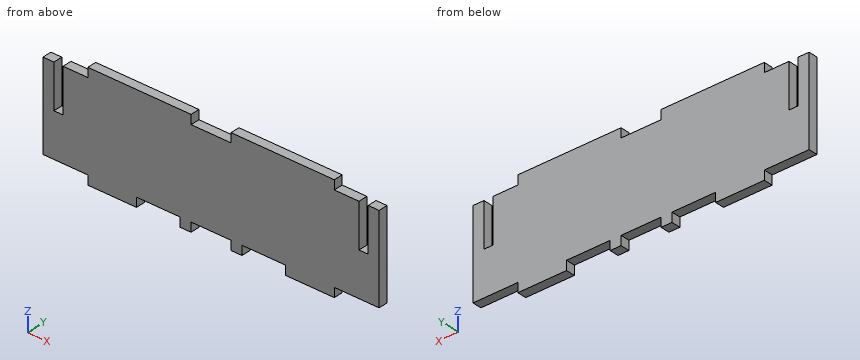
```python
from build123d import *

# Parameters (mm, degrees)
F0_W     = 60.071
F0_H     = 5.334
F0_W_2   = 28.321
F0_W_3   = 6.35
F1_DEPTH = 5.3594


with BuildPart() as f1:
    # F0 (on Front) → F1 (new body)
    with BuildSketch(Plane.XZ):
        with Locations((56.1213, 53.467)):
            Rectangle(F0_W, F0_H)
        with Locations((139.466246, 53.467)):
            Rectangle(F0_W, F0_H)
        Polygon((0, 50.8), (0, 0), (26.0858, 0), (54.4068, 0), (79.8068, 0), (86.1568, 0), (109.430746, 0), (115.780746, 0), (141.180746, 0), (169.501746, 0), (195.587546, 0), (195.587546, 50.8), (189.237546, 50.8), (189.237546, 25.4), (183.903546, 25.4), (183.903546, 50.8), (169.501746, 50.8), (109.430746, 50.8), (86.1568, 50.8), (26.0858, 50.8), (11.684, 50.8), (11.684, 25.4), (6.35, 25.4), (6.35, 50.8), align=None)
        with Locations((40.2463, -2.667)):
            Rectangle(F0_W_2, F0_H)
        with Locations((82.9818, -2.667)):
            Rectangle(F0_W_3, F0_H)
        with Locations((112.605746, -2.667)):
            Rectangle(F0_W_3, F0_H)
        with Locations((155.341246, -2.667)):
            Rectangle(F0_W_2, F0_H)
    extrude(amount=F1_DEPTH)


solid = f1.part
```
The model under review builds one solid part; all positions refer to its coordinate system, in mm. Round coordinates to 2 decimals unless told otherwise and drop trailing zeros. Loops run counter-clockwise (first coordinate to the right, second up) from the corner with the lowest first, then second, coordinate; pieces in that order, holes last. Notation, with made-up numbers: (7.5, -17) - (63.5, -17) arc R24 ccw to (63.5, 1) - close; hole circle Ø2 at (36, 3). An arc over 180 degrees is marked (long way). Write each question's results on one line, items separated by ' | '. Start each with the question number.
Q1. Take a section at A-A on z = 44. Give the boundary of the cut face in (x, y), plus the area to 3 significant figures.
Q2. Wall thickness on line 1 along X through (y, z) = (-0.9, -1); line 2 along X through (y, z) = (-4.8, 48.5); line 3 along Z through (x, y) = (179, -1.45): over which ranges is each line inside the solid? List them lowest first. Write a range as [from, to].
Q3. Take a section at B-B on x = 62. Give the boundary of the cut face in (y, z).
Q4. Insertion check: P1, Ø2.5, axis at x = 69.5, y = -2, coming from the -Z side; P2, Ø1.6, axis at x = 99.5, y = -2, coming from the +Z side; P3, Ø2.5, axis at y = -2, z = 53.5, coming from the -X side. Each pin has a flat end and moves straight along its axis. Give the tip position at first contact, or say it passes through.
Data:
1) outline: (0, -5.36) - (6.35, -5.36) - (6.35, 0) - (0, 0) - close; (11.68, -5.36) - (183.9, -5.36) - (183.9, 0) - (11.68, 0) - close; (189.24, -5.36) - (195.59, -5.36) - (195.59, 0) - (189.24, 0) - close | area: 991 mm²
2) line 1: x = [26.09, 54.41], [79.81, 86.16], [109.43, 115.78], [141.18, 169.5] | line 2: x = [0, 6.35], [11.68, 183.9], [189.24, 195.59] | line 3: z = [0, 50.8]
3) outline: (-5.36, 0) - (0, 0) - (0, 56.13) - (-5.36, 56.13) - close
4) P1: stops at z = 0 | P2: stops at z = 50.8 | P3: stops at x = 26.09
